Check sheet for the drawn part. Datum: minimum x, y, z corner. Units: mm. A direction names the side the tool comes from. Round coordinates to 2 decimals unless told otherwise and drop trailing zeros. Write each loop counter-clockwise with the first axis right and the second up, starting at its lowest first coordinate (ties: lowest second). Pieces come first, ordered by that corner, then holes. Notation, with made-up numbers: M 3.25,49 L 12.25,49 A35 ccw 12.25,81 Z; hole C -4,-6.5 d6. An arc over 180 degrees is marked long. Use a Markdown table: item, result.
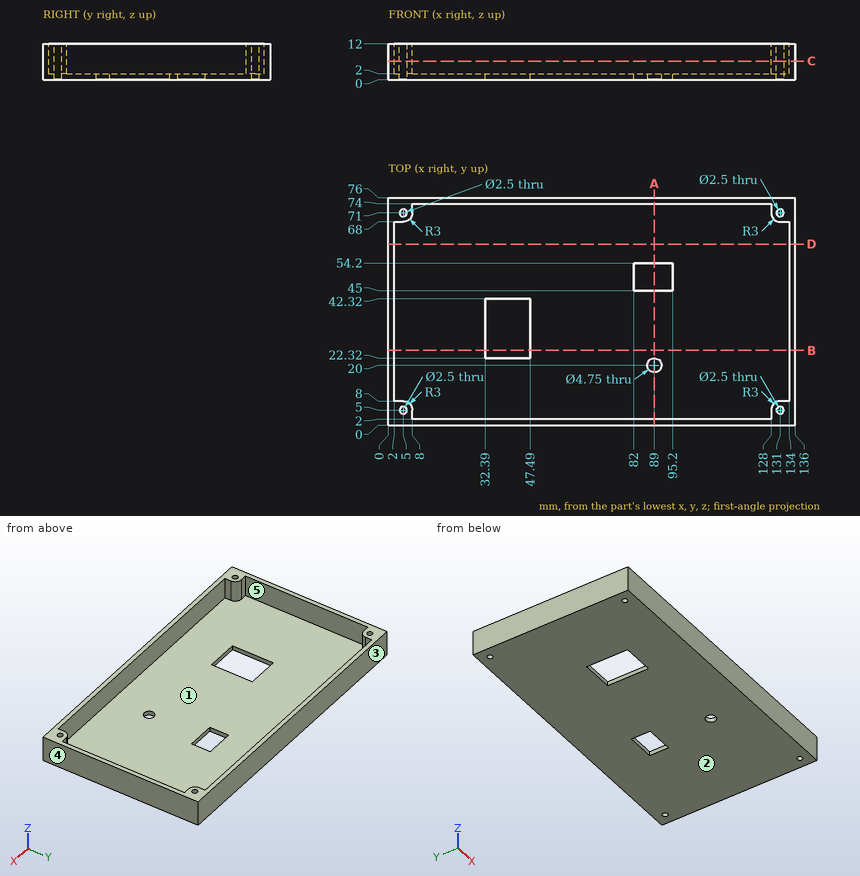
Item 1: Cross-section at D-D, the plane y = 60.5. Record the cut outline in (x, z), and give its area (3 significant figures).
Outcome:
| item | result |
|---|---|
| outline | M 0,0 L 136,0 L 136,12 L 134,12 L 134,2 L 2,2 L 2,12 L 0,12 Z |
| area | 312 mm2 |
Item 2: Cross-section at C-C, the plane z = 6.25. Record the cut outline in (x, y), and give its area (3 significant figures).
Outcome:
| item | result |
|---|---|
| outline | M 0,0 L 136,0 L 136,76 L 0,76 Z; hole M 2,8 L 5,8 A3 cw 8,5 L 8,2 L 128,2 L 128,5 A3 cw 131,8 L 134,8 L 134,68 L 131,68 A3 cw 128,71 L 128,74 L 8,74 L 8,71 A3 cw 5,68 L 2,68 Z; hole C 5,5 d2.5; hole C 5,71 d2.5; hole C 131,5 d2.5; hole C 131,71 d2.5 |
| area | 949 mm2 |
Item 3: Go/stop test with a flat-tipped pin: pin 1 (2 mm diameter, centred on x = 5, y = 71, fed in from -Z). Record where the tip stops, or that it passes through.
Outcome:
| item | result |
|---|---|
| pin 1 | passes through |
Item 4: Material ranges on line 1 along Y through (x, z) = (5, 8); line 2 along X through (y, z) = (46, 1.5); line 3 along X through (y, z) = (31, 2.75), recorded low to high. Write a range as from..to.
Outcome:
| item | result |
|---|---|
| line 1 | y = 0..3.75, 6.25..8, 68..69.75, 72.25..76 |
| line 2 | x = 0..82, 95.2..136 |
| line 3 | x = 0..2, 134..136 |
Item 5: Mould release check, pull along Y, two halves, no side actions. Record for the marked faces 3, 4 and 5: +Y half, -Y half, draft (parallel to the pull), parting line (faces both ways), or undercut.
Outcome:
| item | result |
|---|---|
| face 3 | +Y half |
| face 4 | draft |
| face 5 | undercut |
Item 6: Access from +Z, -Z, +X, -X, +Y, -Y to the whole of each face (thin tool, end or side, straight path). Record for the marked faces 1 and 2.
Outcome:
| item | result |
|---|---|
| face 1 | +Z |
| face 2 | -Z, +X, -X, +Y, -Y |
Item 7: Cross-section at A-A, the plane x = 89. Record the cut outline in (y, z) (3 decimals), and give its area (3 significant figures).
Outcome:
| item | result |
|---|---|
| outline | M 0,0 L 17.625,0 L 17.625,2 L 2,2 L 2,12 L 0,12 Z; M 22.375,0 L 45,0 L 45,2 L 22.375,2 Z; M 54.2,0 L 76,0 L 76,12 L 74,12 L 74,2 L 54.2,2 Z |
| area | 164 mm2 |
Item 8: Cross-section at B-B, the plane y = 25. Record the cut outline in (x, z), and give its area (3 significant figures).
Outcome:
| item | result |
|---|---|
| outline | M 0,0 L 32.39,0 L 32.39,2 L 2,2 L 2,12 L 0,12 Z; M 47.49,0 L 136,0 L 136,12 L 134,12 L 134,2 L 47.49,2 Z |
| area | 282 mm2 |
